from build123d import *

# Parameters (mm, degrees)
SKETCH1_W           = 52
SKETCH1_H           = 38
BOSS_EXTRUDE1_DEPTH = 5
SKETCH2_W           = 52
SKETCH2_H           = 6
BOSS_EXTRUDE2_DEPTH = 23
SKETCH3_R           = 9
CUT_EXTRUDE1_DEPTH  = 6
SKETCH4_R           = 1.15
CUT_EXTRUDE2_DEPTH  = 6
SKETCH5_W           = 6
SKETCH5_H           = 32
BOSS_EXTRUDE3_DEPTH = 23
CUT_EXTRUDE3_DEPTH  = 136.306891562
SKETCH7_R           = 1.65
CUT_EXTRUDE4_DEPTH  = 5
SKETCH8_R           = 1.65
CUT_EXTRUDE5_DEPTH  = 5
SKETCH9_W           = 6
SKETCH9_H           = 4.814654703
CUT_EXTRUDE6_DEPTH  = 1
CHAMFER1_SIZE       = 1
SKETCH10_R          = 2
CUT_EXTRUDE7_DEPTH  = 1


with BuildPart() as part:
    # Sketch1 → Boss-Extrude1 (new body)
    with BuildSketch(Plane.XY):
        with Locations((-57.914180529, 102.737237131)):
            Rectangle(SKETCH1_W, SKETCH1_H)
    extrude(amount=BOSS_EXTRUDE1_DEPTH)

    # Sketch2 → Boss-Extrude2 (add)
    with BuildSketch(Plane.XY.offset(5)):
        with Locations((-57.914180529, 118.737237131)):
            Rectangle(SKETCH2_W, SKETCH2_H)
    extrude(amount=BOSS_EXTRUDE2_DEPTH)

    # Sketch3 → Cut-Extrude1 (cut)
    with BuildSketch(Plane(origin=(0, 121.737237131, 0), x_dir=(1, 0, 0), z_dir=(0, 1, 0))):
        with Locations(Location((-57.914080529, -15.0001, 0), (0, 0, 270))):
            Circle(SKETCH3_R)
    extrude(amount=-CUT_EXTRUDE1_DEPTH, mode=Mode.SUBTRACT)

    # Sketch4 → Cut-Extrude2 (cut)
    with BuildSketch(Plane.XZ.offset(-115.737237131)):
        with Locations(Location((-65.914080529, 23.0001, 0), (0, 0, 270))):
            Circle(SKETCH4_R)
        with Locations(Location((-49.914080529, 23.0001, 0), (0, 0, 270))):
            Circle(SKETCH4_R)
        with Locations(Location((-49.914080529, 7.0001, 0), (0, 0, 270))):
            Circle(SKETCH4_R)
        with Locations(Location((-65.914080529, 7.0001, 0), (0, 0, 270))):
            Circle(SKETCH4_R)
    extrude(amount=-CUT_EXTRUDE2_DEPTH, mode=Mode.SUBTRACT)

    # Sketch5 → Boss-Extrude3 (add)
    with BuildSketch(Plane.XY.offset(5)):
        with Locations((-80.914180529, 99.737237131)):
            Rectangle(SKETCH5_W, SKETCH5_H)
        with Locations((-34.914180529, 99.737237131)):
            Rectangle(SKETCH5_W, SKETCH5_H)
    extrude(amount=BOSS_EXTRUDE3_DEPTH)

    # Sketch6 → Cut-Extrude3 (cut, through all)
    with BuildSketch(Plane.ZY.offset(83.914180529)):
        Polygon((5, 83.737237131), (5, 93.737237131), (28, 115.737237131), (34.8001915, 115.737237131), (34.8001915, 79.151046586), (5, 79.151046586), align=None)
    extrude(amount=-CUT_EXTRUDE3_DEPTH, mode=Mode.SUBTRACT)

    # Sketch7 → Cut-Extrude4 (cut)
    with BuildSketch(Plane.XY.offset(5)):
        with Locations((-42.914180529, 110.737237131)):
            Circle(SKETCH7_R)
        with Locations((-42.914180529, 88.737237131)):
            Circle(SKETCH7_R)
        with Locations((-72.914180529, 110.737237131)):
            Circle(SKETCH7_R)
        with Locations((-72.914180529, 88.737237131)):
            Circle(SKETCH7_R)
    extrude(amount=-CUT_EXTRUDE4_DEPTH, mode=Mode.SUBTRACT)

    # Sketch8 → Cut-Extrude5 (cut)
    with BuildSketch(Plane.XY.offset(5)):
        with Locations((-72.914180529, 99.737237131)):
            Circle(SKETCH8_R)
        with Locations((-42.914180529, 99.737237131)):
            Circle(SKETCH8_R)
    extrude(amount=-CUT_EXTRUDE5_DEPTH, mode=Mode.SUBTRACT)

    # Sketch9 → Cut-Extrude6 (cut)
    with BuildSketch(Plane(origin=(0, 121.737237131, 0), x_dir=(1, 0, 0), z_dir=(0, 1, 0))):
        with Locations((-57.914180529, -25.592672648)):
            Rectangle(SKETCH9_W, SKETCH9_H)
    extrude(amount=-CUT_EXTRUDE6_DEPTH, mode=Mode.SUBTRACT)

    # Chamfer1
    chamfer1_edges = [part.edges().sort_by_distance(p)[0] for p in [
        (-60.914180529, 120.737237131, 25.742673009),
        (-54.914180529, 120.737237131, 25.742708364),
    ]]
    chamfer(chamfer1_edges, length=CHAMFER1_SIZE - 0.0001)  # a hair under: the kernel refuses the full size

    # Sketch10 → Cut-Extrude7 (cut)
    with BuildSketch(Plane(origin=(0, 121.737237131, 0), x_dir=(1, 0, 0), z_dir=(0, 1, 0))):
        with Locations(Location((-65.914080529, -7.0001, 0), (0, 0, 270))):
            Circle(SKETCH10_R)
        with Locations(Location((-49.914080529, -7.0001, 0), (0, 0, 270))):
            Circle(SKETCH10_R)
        with Locations(Location((-49.914080529, -23.0001, 0), (0, 0, 270))):
            Circle(SKETCH10_R)
        with Locations(Location((-65.914080529, -23.0001, 0), (0, 0, 270))):
            Circle(SKETCH10_R)
    extrude(amount=-CUT_EXTRUDE7_DEPTH, mode=Mode.SUBTRACT)


solid = part.part
Part model, mm, in its own coordinate system. A direction names the side the tool comes from. Coordinates: 2 decimals unless noted, no trailing zeros. Loops run counter-clockwise (first coordinate to the right, second up) from the corner with the lowest first, then second, coordinate; pieces in that order, holes last. Notation, with made-up numbers: M 63.25,-3.75 L 118.25,-3.75 A10 cw 118.25,15.25 Z; hole C 5,-1 d4. An arc over 180 degrees is marked long. Use a Markdown table: item, result. Add a question column.
Q1. Cut at A-A (z = 16.75). Write the cut outline in (x, y), and give its area (3 significant figures).
Q2. Probe L1, parallel to Z at x = -58, y = 118; L2, parallel to X at y = 105.5, z = 10; L3, parallel to Y at x = -75.5, z = 18.5. List the from-to ranges inside material, lowest first.
Q3. Pin check, flat tips, straight feed: P1, Ø2, axis at x = -66, z = 22.5, coming from the +Y side; P2, Ø5, axis at x = -65.91, z = 23, coming from the -Y side; P3, Ø2, axis at x = -78, y = 100.5, coming from the +Z side. Stop position of each tip, or through.
Q4. Mould opens along X. For faces 1 (the flat face through (-58, 100, 5)), 2 (the flat face through (-83.914, 107, 11)), 3 (the flat face through (-58, 119, 28)) say: +X half, -X half, draft (parallel to the pull), parting line (faces both ways), or undercut.
Q5. Which spindle directions (+Z, -Z, +X, -X, +Y, -Y) get a long thin tool onto all of the face, cutting with end or side? Do faces 4 (the flat face through (-58, 120.737, 26)), 5 (the cylindrical face through (-67.13, 121.24, 21.41)), 6 (the flat face through (-37.914, 109, 11)). Say none if no direction does.
Q6. Cut at C-C (z = 2.75). Write the cut outline in (x, y).
Q7. Cut at B-B (x = -63). Write the cut outline in (y, z).
Q8. Cut at D-D (y = 113.5). Write the cut outline in (x, z).
Worked out:
| question | item | result |
|---|---|---|
| 1 | outline | M -83.91,104.98 L -77.91,104.98 L -77.91,115.74 L -66.74,115.74 L -66.74,121.74 L -83.91,121.74 Z; M -49.09,115.74 L -37.91,115.74 L -37.91,104.98 L -31.91,104.98 L -31.91,121.74 L -49.09,121.74 Z |
| 1 | area | 335 mm2 |
| 2 | L1 | z = 0 to 6, 24 to 28 |
| 2 | L2 | x = -83.91 to -77.91, -37.91 to -31.91 |
| 2 | L3 | y = 115.74 to 121.74 |
| 3 | P1 | stops at y = 120.74 |
| 3 | P2 | stops at y = 115.74 |
| 3 | P3 | stops at z = 13.12 |
| 4 | face 1 | undercut |
| 4 | face 2 | -X half |
| 4 | face 3 | draft |
| 5 | face 4 | +Z, +Y |
| 5 | face 5 | +Y |
| 5 | face 6 | +Z, -Y |
| 6 | outline | M -83.91,83.74 L -31.91,83.74 L -31.91,121.74 L -83.91,121.74 Z; hole C -72.91,88.74 d3.3; hole C -72.91,99.74 d3.3; hole C -72.91,110.74 d3.3; hole C -42.91,88.74 d3.3; hole C -42.91,99.74 d3.3; hole C -42.91,110.74 d3.3 |
| 7 | outline | M 83.74,0 L 121.74,0 L 121.74,7.57 L 115.74,7.57 L 115.74,5 L 83.74,5 Z; M 115.74,22.43 L 121.74,22.43 L 121.74,28 L 115.74,28 Z |
| 8 | outline | M -83.91,0 L -31.91,0 L -31.91,25.66 L -37.91,25.66 L -37.91,5 L -77.91,5 L -77.91,25.66 L -83.91,25.66 Z |
